Build history of the part. All positions in model axes, mm. Face numbers are marked on the shaded views. A direction names the side the tool comes from. Give positions to 0.01 mm unless a question says otherwise; leave off trailing zeros. Loops run counter-clockwise (first coordinate to the right, second up) from the corner with the lowest first, then second, coordinate; pieces in that order, holes last.
1) Band-saw the part on B-B on x = -29. List the corners of the cut face in (y, z), then the cut area to 3 significant figures.
2) Band-saw the part on A-A on y = 50.5. List the corners of the cut face in (x, z), then the cut area to 3 significant figures.
3) Band-saw the part on C-C on z = -35. List the corners of the cut face in (x, y).
4) 3-axis set-ups, long thin cutter, end or side, ignore diameter. For the marked faces 1 and 2: which of +Z, -Z, +X, -X, +Y, -Y reach the whole face in a straight line?
5) Two-plate mould, pull along X, no slides. Class the marked faces 3, 4, 5 and 6: +X half, -X half, draft (parallel to the pull), parting line (faces both ways), or undercut.
6) Flat gauge pins, fed straight in: P1, Ø6, axis at x = 57.51, z = 57.51, coming from the +Y side; P2, Ø1.5, axis at x = 73.5, y = 46.5, coming from the -Z side; P3, Ø2.5, axis at y = 37, z = -74, coming from the -X side. Where does each tip first touch, or does it go through?
7) Wall check: line 1 (Z direction, x = -28, y = 15.5); line 2 (Y direction, x = 60, z = 65.5). Give the ranges that are in metal, low to high.
8) Band-saw the part on D-D on x = 46.5. List the corners of the cut face in (y, z), then the cut area to 3 significant figures.
```python
from build123d import *

# Parameters (mm, degrees)
SKETCH2_W           = 150
SKETCH2_H           = 150
BOSS_EXTRUDE1_DEPTH = 85
SHELL1_T            = -3
CUT_EXTRUDE1_DEPTH  = 82
CUT_EXTRUDE2_DEPTH  = 4
SKETCH5_R           = 2.5
CUT_EXTRUDE3_DEPTH  = 4


with BuildPart() as part:
    # Sketch2 → Boss-Extrude1 (new body)
    with BuildSketch(Plane(origin=(0, 0, 0), x_dir=(1, 0, 0), z_dir=(0, 1, 0))):
        Rectangle(SKETCH2_W, SKETCH2_H)
    extrude(amount=BOSS_EXTRUDE1_DEPTH)

    # Shell1
    shell1_openings = [part.faces().sort_by_distance(p)[0] for p in [
        (0, 85, 0),
    ]]
    offset(amount=SHELL1_T, openings=shell1_openings, kind=Kind.INTERSECTION)

    # Sketch3 → Cut-Extrude1 (cut)
    with BuildSketch(Plane(origin=(0, 85, 0), x_dir=(1, 0, 0), z_dir=(0, 1, 0))):
        Polygon((39.644660941, -75), (75, -75), (75, -39.644660941), (72, -39.644660941), (72, -42.644660941), (72, -72), (39.644660941, -72), align=None)
        Polygon((-39.644660941, -72), (-42.644660941, -72), (-72, -72), (-72, -39.644660941), (-75, -39.644660941), (-75, -75), (-39.644660941, -75), align=None)
        Polygon((-72, 39.644660941), (-72, 42.644660941), (-72, 72), (-39.644660941, 72), (-39.644660941, 75), (-75, 75), (-75, 39.644660941), align=None)
        Polygon((39.644660941, 72), (42.644660941, 72), (72, 72), (72, 39.644660941), (75, 39.644660941), (75, 75), (39.644660941, 75), align=None)
    extrude(amount=-CUT_EXTRUDE1_DEPTH, mode=Mode.SUBTRACT)

    # Sketch4 → Cut-Extrude2 (cut, through all)
    with BuildSketch(Plane(origin=(0, 3, 0), x_dir=(1, 0, 0), z_dir=(0, 1, 0))):
        Polygon((-75, -57.32233047), (-75, -75), (-57.32233047, -75), align=None)
        Polygon((-75, 57.32233047), (-57.32233047, 75), (-75, 75), align=None)
        Polygon((57.32233047, 75), (75, 57.32233047), (75, 75), align=None)
        Polygon((75, -57.32233047), (57.32233047, -75), (75, -75), align=None)
    extrude(amount=-CUT_EXTRUDE2_DEPTH, mode=Mode.SUBTRACT)

    # Sketch5 → Cut-Extrude3 (cut, through all)
    with BuildSketch(Plane(origin=(0, 3, 0), x_dir=(1, 0, 0), z_dir=(0, 1, 0))):
        with Locations((57.511546526, 57.511546526)):
            Circle(SKETCH5_R)
        with Locations((57.511546526, -57.511546526)):
            Circle(SKETCH5_R)
        with Locations((-57.511546526, -57.511546526)):
            Circle(SKETCH5_R)
        with Locations((-57.511546526, 57.511546526)):
            Circle(SKETCH5_R)
    extrude(amount=-CUT_EXTRUDE3_DEPTH, mode=Mode.SUBTRACT)


solid = part.part
```
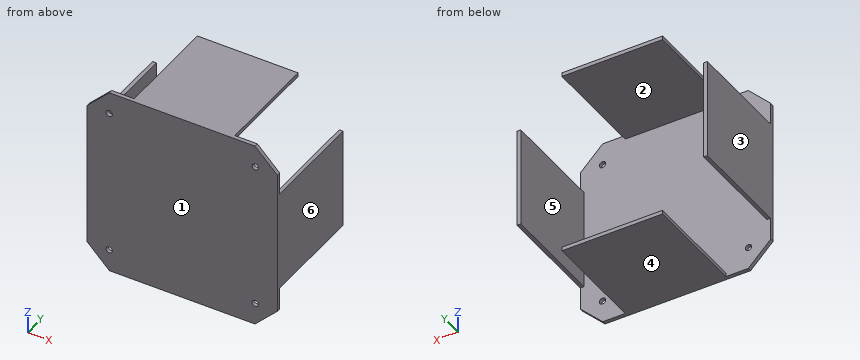
Findings below:
1. outline: (0, -75) - (85, -75) - (85, -72) - (3, -72) - (3, 72) - (85, 72) - (85, 75) - (0, 75) - close
1. area: 942 mm2
2. outline: (-75, -39.64) - (-72, -39.64) - (-72, 39.64) - (-75, 39.64) - close; (-39.64, -75) - (39.64, -75) - (39.64, -72) - (-39.64, -72) - close; (-39.64, 72) - (39.64, 72) - (39.64, 75) - (-39.64, 75) - close; (72, -39.64) - (75, -39.64) - (75, 39.64) - (72, 39.64) - close
2. area: 951 mm2
3. outline: (-75, 0) - (75, 0) - (75, 85) - (72, 85) - (72, 3) - (-72, 3) - (-72, 85) - (-75, 85) - close
4. face 1: +Z, -Z, +X, -X, -Y
4. face 2: +X, -X, +Y
5. face 3: -X half
5. face 4: draft
5. face 5: undercut
5. face 6: +X half
6. P1: stops at y = 3
6. P2: stops at z = -39.64
6. P3: stops at x = -39.64
7. line 1: z = -75 to -72, 72 to 75
7. line 2: y = 0 to 3
8. outline: (0, -75) - (3, -75) - (3, 75) - (0, 75) - close
8. area: 450 mm2
